```python
from build123d import *

# Parameters (mm, degrees)
SKETCH1_W               = 50
SKETCH1_H               = 50
BOSS_EXTRUDE1_DEPTH     = 100
CUT_EXTRUDE1_DEPTH      = 4.5
SKETCH4_R               = 2.5
BOSS_EXTRUDE2_DEPTH     = 4.5
CUT_EXTRUDE2_DEPTH      = 159.730116865
CUT_EXTRUDE2_DEPTH_BACK = 159.730116865
FILLET1_R               = 10


with BuildPart() as part:
    # Sketch1 → Boss-Extrude1 (new body)
    with BuildSketch(Plane(origin=(0, 0, 0), x_dir=(1, 0, 0), z_dir=(0, 1, 0))):
        Rectangle(SKETCH1_W, SKETCH1_H)
    extrude(amount=BOSS_EXTRUDE1_DEPTH)

    # Sketch2 → Cut-Extrude1 (cut)
    with BuildSketch(Plane.XY.offset(25)):
        with BuildLine():
            Line((-25, 0), (25, 0))
            Line((25, 0), (25, 21))
            Line((25, 21), (24.269322199, 21))
            ThreePointArc((24.269322199, 21), (0, 40), (-24.269322199, 21))
            Line((-24.269322199, 21), (-25, 21))
            Line((-25, 21), (-25, 0))
        make_face()
    cut_extrude1 = extrude(amount=-CUT_EXTRUDE1_DEPTH, mode=Mode.SUBTRACT)

    # Mirror1: Cut-Extrude1 across plane
    add(cut_extrude1.mirror(Plane.XY), mode=Mode.SUBTRACT)

    # Sketch4 → Boss-Extrude2 (add)
    with BuildSketch(Plane(origin=(0, 0, -25), x_dir=(-1, 0, 0), z_dir=(0, 0, -1))):
        with BuildLine():
            Line((-25, 100), (25, 100))
            Line((25, 100), (25, 125))
            ThreePointArc((25, 125), (0, 150), (-25, 125))
            Line((-25, 125), (-25, 100))
        make_face()
        with Locations((0, 125)):
            Circle(SKETCH4_R, mode=Mode.SUBTRACT)
    boss_extrude2 = extrude(amount=-BOSS_EXTRUDE2_DEPTH)

    # Mirror2: Boss-Extrude2 across plane
    add(boss_extrude2.mirror(Plane.XY))

    # Sketch5 → Cut-Extrude2 (cut, two sides: drawn at the far end of the back side and taken through both)
    with BuildSketch(Plane(origin=(0, 0, -20.5), x_dir=(-1, 0, 0), z_dir=(0, 0, -1)).offset(-CUT_EXTRUDE2_DEPTH_BACK)):
        with BuildLine():
            Line((-25, 15), (-25, -11.716119479))
            Line((-25, -11.716119479), (25, -11.716119479))
            Line((25, -11.716119479), (25, 15))
            ThreePointArc((25, 15), (0, -10), (-25, 15))
        make_face()
    extrude(amount=CUT_EXTRUDE2_DEPTH + CUT_EXTRUDE2_DEPTH_BACK, mode=Mode.SUBTRACT)

    # Fillet1
    fillet1_edges = [part.edges().sort_by_distance(p)[0] for p in [
        (20, 0, 0),
        (-20, 0, 0),
    ]]
    fillet(fillet1_edges, radius=FILLET1_R)


solid = part.part
```
The listing builds one solid part. Answer for the finished solid, in the listing's coordinates (mm). A direction names the side the tool comes from. Round coordinates to 2 decimals unless told otherwise and drop trailing zeros. Write each loop counter-clockwise with the first axis right and the second up, starting at its lowest first coordinate (ties: lowest second). Pieces come first, ordered by that corner, then holes. Notation, with made-up numbers: (-1.75, 1) -> (44.25, 1) arc R29 ccw to (44.25, 26) -> close; hole circle Ø5 at (65, -26.75). An arc over 180 degrees is marked (long way). Use CSV: the item, a comma, the result in double quotes. Start each with the question number.
(1) Section D-D on y = 137.5 is taken. Give the vertices of the cut face in (x, z), then the cut area to 3 significant figures.
(2) Section B-B on y = 117 is taken. Give the vertices of the cut face in (x, z), then the cut area to 3 significant figures.
(3) Each of these flat-tipped pins is pushed along its axis until it touches: pin 1 (1.5 mm diameter, centred on x = -6.5, z = -4.5, fed in from +Y); pin 2 (0.8 mm diameter, centred on x = 24.5, z = -24, fed in from -Y); pin 3 (2 mm diameter, centred on x = 18, z = 0, fed in from -Y). Where does it stop, or does it pass through?
(4) Which of the six approach directions +Z, -Z, +X, -X, +Y, -Y give full straight-line access (tool end or side, diameter ignored) to faces 4 (the face through (0, 40, -23)), 5 (the face through (0, 40, 23)), 6 (the face through (0, 120, 20.5))?
(5) Section A-A on x = 0 is taken. Give the vertices of the cut face in (y, z).
(6) Consider L1, parallel to Z at x = 3.5, y = 125; L2, parallel to Y at x = 0, z = -22.8; L3, parallel to Z at x = -18, y = 27.5. Determine where each line is inside the solid, lowest interval first. Write a range as from..to.
(7) The mould has two halves that part along Y. Classify faces 1 (the face through (-24.65, 10.83, 0.29)), 2 (the face through (0.33, 127.48, -22.78)), 3 (the face through (0, 120, -20.5)): released by +Y, released by -Y, zero draft, split by the parting line, or undercut.
(8) Section C-C on z = 22 is taken. Give the vertices of the cut face in (x, y).
A:
1,outline,"(-21.65, -25) -> (21.65, -25) -> (21.65, -20.5) -> (-21.65, -20.5) -> close; (-21.65, 20.5) -> (21.65, 20.5) -> (21.65, 25) -> (-21.65, 25) -> close"
1,area,"390 mm²"
2,outline,"(-25, -25) -> (25, -25) -> (25, -20.5) -> (-25, -20.5) -> close; (-25, 20.5) -> (25, 20.5) -> (25, 25) -> (-25, 25) -> close"
2,area,"450 mm²"
3,pin 1,"stops at y = 100"
3,pin 2,"stops at y = 21"
3,pin 3,"stops at y = 0.42"
4,face 4,"-Z, -Y"
4,face 5,"+Z, -Y"
4,face 6,"+X, -X, +Y"
5,outline,"(0, -20.5) -> (40, -20.5) -> (40, -25) -> (122.5, -25) -> (122.5, -20.5) -> (100, -20.5) -> (100, 20.5) -> (122.5, 20.5) -> (122.5, 25) -> (40, 25) -> (40, 20.5) -> (0, 20.5) -> close; (127.5, -25) -> (150, -25) -> (150, -20.5) -> (127.5, -20.5) -> close; (127.5, 20.5) -> (150, 20.5) -> (150, 25) -> (127.5, 25) -> close"
6,L1,"z = -25..-20.5, 20.5..25"
6,L2,"y = 40..122.5, 127.5..150"
6,L3,"z = -20.5..20.5"
7,face 1,"released by -Y"
7,face 2,"undercut"
7,face 3,"zero draft"
8,outline,"(-25, 21) -> (-24.27, 21) arc R25 cw to (24.27, 21) -> (25, 21) -> (25, 125) arc R25 ccw to (-25, 125) -> close; hole circle Ø5 at (0, 125)"
